Design review of the part shown in the three views and the two pictorial views. Dimensions are in mm from the part's minimum x, y and z. A direction names the side the tool comes from. Round coordinates to 2 decimals unless told otherwise and drop trailing zeros. Order: outer loops, then holes, each group sorted by start corner. A loop starts at its lowest first (then second) coordinate and runs counter-clockwise, first axis right, second up. Notation, with made-up numbers: M 53.5,-36 L 108.5,-36 A16 ccw 108.5,-23 Z; hole C 34.25,15.25 d6. An arc over 180 degrees is marked long. Use a Markdown table: item, result. Add a question column.
(1) Machinability: for the marked faces 1 and 2, which of the approach directions +Z, -Z, +X, -X, +Y, -Y give a long, thin tool a straight path to every point of the face, cutting with its end or side? Answer none if there is none.
(2) Take a section at B-B (x = 36.25). Write out the cut boundary in (y, z), then the cut area to 3 significant figures.
(3) Take a section at C-C (z = 11.5). Write out the cut boundary in (x, y), then the cut area to 3 significant figures.
(4) The part is to be moulded in two halves that separate along Z. For the marked faces 3, 4 and 5, say which applies: released by +Z, released by -Z, zero draft, split by the parting line, or undercut.
(5) To check wall thickness, follow probe 1 along Y at (x, z) = (36.25, 14); probe 2 along X at (y, z) = (32.5, 12.25); probe 3 along Y at (x, z) = (7, 5). State the ranges of each line that lie inside material, in increasing order. Write a range as from..to.
(6) Take a section at A-A (y = 5). Write out the cut boundary in (x, z), then the cut area to 3 significant figures.
(7) Take a section at D-D (z = 25.75). Write out the cut boundary in (x, y), then the cut area to 3 significant figures.
(8) For pin 1 (5.5 mm diameter, centred on x = 36.25, y = 5, fed in from -Z), flat-tipped, find the tip position at first contact; note if it passes through.
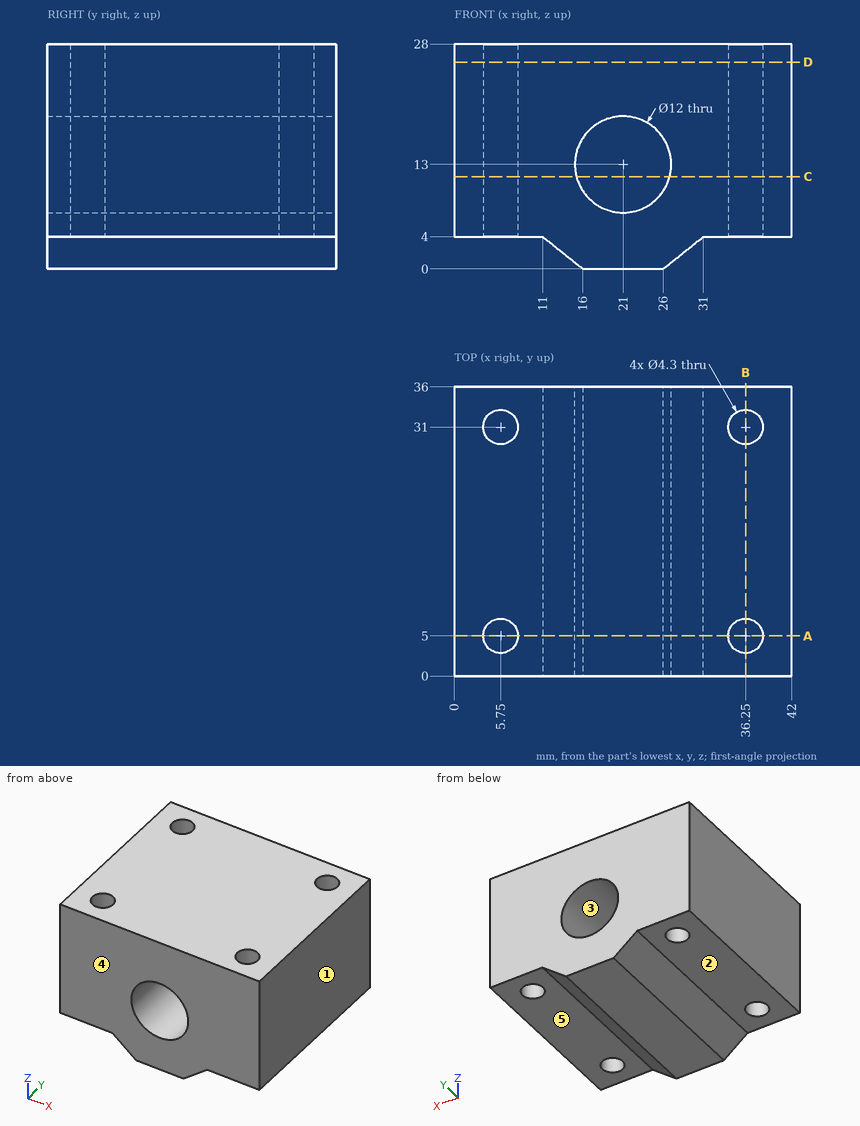
Verdict:
| question | item | result |
|---|---|---|
| 1 | face 1 | +Z, -Z, +X, +Y, -Y |
| 1 | face 2 | -Z, -X, +Y, -Y |
| 2 | outline | M 0,4 L 2.85,4 L 2.85,28 L 0,28 Z; M 7.15,4 L 28.85,4 L 28.85,28 L 7.15,28 Z; M 33.15,4 L 36,4 L 36,28 L 33.15,28 Z |
| 2 | area | 658 mm^2 |
| 3 | outline | M 0,0 L 15.19,0 L 15.19,36 L 0,36 Z; M 26.81,0 L 42,0 L 42,36 L 26.81,36 Z; hole C 5.75,5 d4.3; hole C 5.75,31 d4.3; hole C 36.25,5 d4.3; hole C 36.25,31 d4.3 |
| 3 | area | 1,040 mm^2 |
| 4 | face 3 | undercut |
| 4 | face 4 | zero draft |
| 4 | face 5 | released by -Z |
| 5 | probe 1 | y = 0..2.85, 7.15..28.85, 33.15..36 |
| 5 | probe 2 | x = 0..4.21, 7.29..15.05, 26.95..34.71, 37.79..42 |
| 5 | probe 3 | y = 0..3.25, 6.75..29.25, 32.75..36 |
| 6 | outline | M 0,4 L 3.6,4 L 3.6,28 L 0,28 Z; M 7.9,4 L 11,4 L 16,0 L 26,0 L 31,4 L 34.1,4 L 34.1,28 L 7.9,28 Z; M 38.4,4 L 42,4 L 42,28 L 38.4,28 Z; hole C 21,13 d12 |
| 6 | area | 749 mm^2 |
| 7 | outline | M 0,0 L 42,0 L 42,36 L 0,36 Z; hole C 5.75,5 d4.3; hole C 5.75,31 d4.3; hole C 36.25,5 d4.3; hole C 36.25,31 d4.3 |
| 7 | area | 1,450 mm^2 |
| 8 | pin 1 | stops at z = 4 |
